Verification items for the finished model (mm, model axes). Coordinates: 2 decimals unless noted, no trailing zeros. Order: outer loops, then holes, each group sorted by start corner. A loop starts at its lowest first (then second) coordinate and runs counter-clockwise, first axis right, second up. Notation, with made-up numbers: M -28,1.5 L 25,1.5 A27 cw 25,24.5 Z; hole C -23,43 d8. An arc over 180 degrees is marked long. Return JSON: item names as keys, results as strings. Group by question number.
Q1. Thickness scan on probe 1 along Z at (x, y) = (-25.5, -17); probe 2 along Y at (x, z) = (-26.5, -34). Record the ranges inside material, lowest first.
Q2. Section check B-B, the plane y = -16.25. Enter the section's corners in (x, z), then the cut area to 3 significant figures.
Q3. Section check A-A, the plane x = 18. Enter the section's corners in (y, z).
Q4. Go/stop test with a flat-tipped pin: pin 1 Ø6.5 at (x, y) = (-4, -16) entering from -Z. Record where the tip stops, or that it passes through.
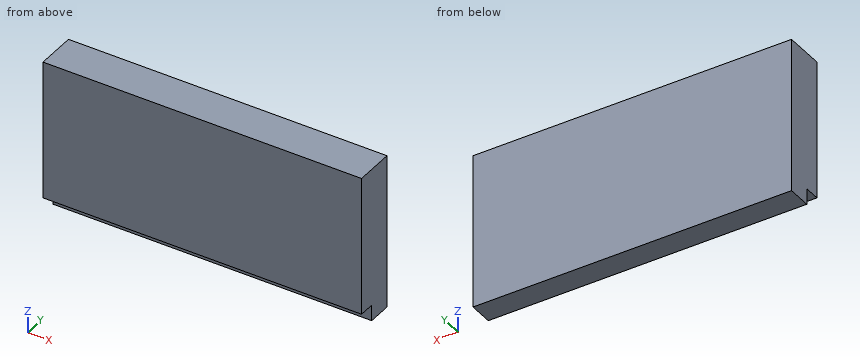
from build123d import *

# Parameters (mm, degrees)
F0_W     = 160
F0_H     = 70
F1_DEPTH = 20
F0_H_2   = 8
F2_DEPTH = 12


with BuildPart() as f1:
    # F0 (on Front) → F1 (new body)
    with BuildSketch(Plane.XZ):
        with Locations((0, 4)):
            Rectangle(F0_W, F0_H)
    extrude(amount=F1_DEPTH)

    # F0 (on Front) → F2 (join)
    with BuildSketch(Plane.XZ):
        with Locations((0, 4)):
            Rectangle(F0_W, F0_H)
        with Locations((0, -35)):
            Rectangle(F0_W, F0_H_2)
    extrude(amount=F2_DEPTH)


solid = f1.part
Numbers:
{
 "1": {"probe 1": "z = -31 to 39", "probe 2": "y = -12 to 0"},
 "2": {"outline": "M -80,-31 L 80,-31 L 80,39 L -80,39 Z", "area": "11,200 mm2"},
 "3": {"outline": "M -20,-31 L -12,-31 L -12,-39 L 0,-39 L 0,39 L -20,39 Z"},
 "4": {"pin 1": "stops at z = -31"}
}
